Can you work these out from the model? Positions are in its coordinate system, mm. Face numbers are marked on the shaded views. Give positions to 0.01 mm unless a question says otherwise; leave off trailing zeros. Order: outer loops, then holes, each group sorted by start corner. A loop starts at its lowest first (then second) coordinate and runs counter-clockwise, first axis right, second up. Notation, with made-up numbers: (-15, 4.5) - (18, 4.5) arc R23 cw to (18, 28.5) - close; hole circle Ø11 at (-36.75, 0). An arc over 180 degrees is marked (long way). Answer as a JSON object with one key per item and string values.
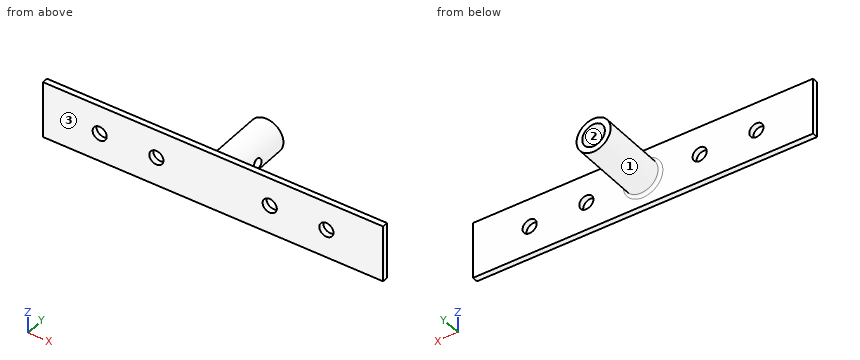
Autodesk Inventor part; units mm, degrees
ref_plane "Work Plane1" through (6, 2, 0) normal (1, 0, 0) x (0, 0, -1)
ref_plane "YZ Plane" through (0, 0, 0) normal (1, 0, 0) x (0, 1, 0)
ref_plane "XZ Plane" through (0, 0, 0) normal (0, 1, 0) x (-1, 0, 0)
sketch "Sketch1" plane through (0, 0, 0) normal (0, 1, 0) x (-1, 0, 0)
  line L0 (60, 10) -> (-60, 10)
  line L1 (-60, 10) -> (-60, -10)
  line L2 (-60, -10) -> (60, -10)
  line L3 (60, -10) -> (60, 10)
  line L4 (60, 10) -> (-60, -10) construction
  line L5 (-60, 10) -> (60, -10) construction
  line L6 (0, 0) -> (20, 0)
  line L7 (20, 0) -> (40, 0)
  line L8 (0, 0) -> (-20, 0)
  line L9 (-20, 0) -> (-40, 0)
  circle A0 centre (-20, 0) radius 2.5
  circle A1 centre (-40, 0) radius 2.5
  circle A2 centre (20, 0) radius 2.5
  circle A3 centre (40, 0) radius 2.5
  dimension "d0" = 120
  dimension "d1" = 20
  dimension "d2" = 20
  dimension "d3" = 20
  dimension "d4" = 20
  dimension "d5" = 20
  dimension "d6" = 5
  dimension "d7" = 5
  dimension "d8" = 5
  dimension "d9" = 5
extrude "Extrusion1" add sketch "Sketch1" along normal blind 2
sketch "Sketch2" plane through (0, 2, 0) normal (0, 1, 0) x (1, 0, 0)
  circle A0 centre (0, 0) radius 4
  circle A1 centre (0, 0) radius 6
  dimension "d12" = 8
  dimension "d13" = 12
extrude "Extrusion2" add sketch "Sketch2" along normal blind 25
fillet "Fillet1" radius 1 1 edges at (-6, 2, 0)
ref_plane "Work Plane1" through (6, 2, 0) normal (1, 0, 0) x (0, 0, -1)
sketch "Sketch3" plane through (6, 2, 0) normal (1, 0, 0) x (0, 0, -1)
  line L0 (0, 0) -> (0, 12)
  circle A0 centre (0, 12) radius 2
  point P0 (0, -2)
  dimension "d17" = 12
  dimension "d18" = 4
extrude "Extrusion3" cut sketch "Sketch3" against normal blind 5
thread "Thread1"
properties part number "2020_ax_connector" material "Aluminum 6061"
Q1. If we section it at A-A, the plane x = 18.5: Please give me the cut outline in (y, z).
Recorded:
{"outline": "(0, -10) - (2, -10) - (2, -2) - (0, -2) - close; (0, 2) - (2, 2) - (2, 10) - (0, 10) - close"}
Q2. If we section it at B-B, the plane z = 0: Count the separate pieces of the cut face and the enclosed holes in it, then the cut area to 3 significant figures.
Recorded:
{"separate pieces": "6", "enclosed holes": "0", "area": "292 mm^2"}
Q3. If we section it at D-D, the plane y = 18.5: Please give me the cut outline in (x, z), then the cut area to 3 significant figures.
Recorded:
{"outline": "circle Ø12 at (0, 0); hole circle Ø8 at (0, 0)", "area": "62.8 mm^2"}
Q4. We'd pull the mould along X, two halves only. Please class the marked faces 1, 2 and 3: released by +X, released by -X, zero draft, split by the parting line, or undercut.
Recorded:
{"face 1": "split by the parting line", "face 2": "undercut", "face 3": "zero draft"}
Q5. I need wall thicknesses on L1, parallel to Z at x = 40, y = 0.7; L2, parallel to Z at x = 0, y = 13.5. Which ranges of each line are inside material? Lowest first, please.
Recorded:
{"L1": "z = -10 to -2.5, 2.5 to 10", "L2": "z = -6 to -4, 4 to 6"}
Q6. I'm going to push flat-ended pins straight in: pin 1 Ø4.5 at (x, z) = (20, 0) entering from +Y; pin 2 Ø8 at (y, z) = (23, -4) entering from +X; pin 3 Ø8 at (y, z) = (14, 7) entering from -X; pin 4 Ø1 at (y, z) = (14, 4.5) entering from +X. Where does each tip first touch, or does it pass through?
Recorded:
{"pin 1": "passes through", "pin 2": "stops at x = 6", "pin 3": "stops at x = -5.2", "pin 4": "stops at x = 4.47"}
Q7. If we section it at C-C, the plane x = 0: Please give me the cut outline in (y, z), then the cut area to 3 significant figures.
Recorded:
{"outline": "(0, -10) - (2, -10) - (2, -7) arc R1 cw to (3, -6) - (27, -6) - (27, -4) - (2, -4) - (2, 4) - (27, 4) - (27, 6) - (3, 6) arc R1 cw to (2, 7) - (2, 10) - (0, 10) - close", "area": "140 mm^2"}
